Autodesk Inventor part; units mm, degrees
ref_plane "YZ Plane" through (0, 0, 0) normal (1, 0, 0) x (0, 1, 0)
ref_plane "XZ Plane" through (0, 0, 0) normal (0, 1, 0) x (-1, 0, 0)
ref_plane "XY Plane" through (0, 0, 0) normal (0, 0, 1) x (1, 0, 0)
sketch "Skizze1" plane through (0, 0, 0) normal (0, 0, 1) x (1, 0, 0)
  line L0 (21, 24.1) -> (-21, 24.1)
  line L1 (-21, 24.1) -> (-21, -21.2)
  line L2 (-21, -21.2) -> (21, -21.2)
  line L3 (21, -21.2) -> (21, 24.1)
  line L4 (10.45, 2) -> (14.55, 2)
  line L5 (14.55, 2) -> (14.55, -2)
  line L6 (14.55, -2) -> (10.45, -2)
  line L7 (10.45, -2) -> (10.45, 2)
  circle A0 centre (12.5, -16) radius 2
  circle A1 centre (-12.5, 16) radius 2
  line L8 (-10.45, 2) -> (-14.55, 2)
  line L9 (-14.55, 2) -> (-14.55, -2)
  line L10 (-14.55, -2) -> (-10.45, -2)
  line L11 (-10.45, -2) -> (-10.45, 2)
  line L12 (12.5, 2) -> (12.5, -2) construction
  line L13 (-12.5, 2) -> (-12.5, -2) construction
  line L14 (14.55, 0) -> (-14.55, 0) construction
  line L15 (0, 0) -> (0, 31.6148) construction
  dimension "d1" = 42
  dimension "d3" = 4
  dimension "d4" = 4
  dimension "d5" = 16
  dimension "d6" = 16
  dimension "d7" = 4
  dimension "d8" = 4.1
  dimension "d9" = 21.2
  dimension "d12" = 25
  dimension "d13" = 24.1
extrude "Extrusion1" add sketch "Skizze1" along normal blind 1.6
properties part number "Platine"
The listing builds one solid part. Answer for the finished solid, in the listing's coordinates (mm). A direction names the side the tool comes from. Round coordinates to 2 decimals unless told otherwise and drop trailing zeros. Loops run counter-clockwise (first coordinate to the right, second up) from the corner with the lowest first, then second, coordinate; pieces in that order, holes last.
Q1. Section D-D, the plane y = -1.5 is taken. Determine the outline of the cut face in (x, z).
Q2. Which of the six approach directions +Z, -Z, +X, -X, +Y, -Y give full straight-line access (tool end or side, diameter ignored) to faces 1 (the face through (12, 2, 1)), 2 (the face through (0, 24.1, 1))?
Q3. For a pull along X with two mould halves and no side action, classify faces 3 (the face through (-21, 2, 1)), 4 (the face through (-14.55, 0, 1)), 5 (the face through (14.55, 0, 1)), 6 (the face through (0, 2, 0)) as released by +X, released by -X, zero draft, split by the parting line, or undercut.
Q4. Section A-A, the plane x = 12.5 is taken. Determine the outline of the cut face in (y, z), then the cut area to 3 significant figures.
Q5. Section B-B, the plane y = 16 is taken. Determine the outline of the cut face in (x, z), then the cut area to 3 significant figures.
Q6. Find the intervals of material crossed by line 1 (Y direction, x = -12.5, z = 1.2); line 2 (Y direction, x = 12.5, z = 0.7); line 3 (X direction, y = 1.5, z = 1.15), in increasing order.
Q7. Section C-C, the plane z = 0.4 is taken. Determine the outline of the cut face in (x, y), then the cut area to 3 significant figures.
Q8. Given pin 1 Ø3 at (x, y) = (12.5, -16) entering from -Z, flat-ended and moving along its own axis, determine where the tip first touches the part or whether it passes through.
Completed:
1. outline: (-21, 0) - (-14.55, 0) - (-14.55, 1.6) - (-21, 1.6) - close; (-10.45, 0) - (10.45, 0) - (10.45, 1.6) - (-10.45, 1.6) - close; (14.55, 0) - (21, 0) - (21, 1.6) - (14.55, 1.6) - close
2. face 1: +Z, -Z
2. face 2: +Z, -Z, +X, -X, +Y
3. face 3: released by -X
3. face 4: undercut
3. face 5: undercut
3. face 6: zero draft
4. outline: (-21.2, 0) - (-18, 0) - (-18, 1.6) - (-21.2, 1.6) - close; (-14, 0) - (-2, 0) - (-2, 1.6) - (-14, 1.6) - close; (2, 0) - (24.1, 0) - (24.1, 1.6) - (2, 1.6) - close
4. area: 59.7 mm2
5. outline: (-21, 0) - (-14.5, 0) - (-14.5, 1.6) - (-21, 1.6) - close; (-10.5, 0) - (21, 0) - (21, 1.6) - (-10.5, 1.6) - close
5. area: 60.8 mm2
6. line 1: y = -21.2 to -2, 2 to 14, 18 to 24.1
6. line 2: y = -21.2 to -18, -14 to -2, 2 to 24.1
6. line 3: x = -21 to -14.55, -10.45 to 10.45, 14.55 to 21
7. outline: (-21, -21.2) - (21, -21.2) - (21, 24.1) - (-21, 24.1) - close; hole (-14.55, -2) - (-10.45, -2) - (-10.45, 2) - (-14.55, 2) - close; hole circle Ø4 at (-12.5, 16); hole (10.45, -2) - (14.55, -2) - (14.55, 2) - (10.45, 2) - close; hole circle Ø4 at (12.5, -16)
7. area: 1,840 mm2
8. pin 1: passes through
